The listing builds one solid part. Answer for the finished solid, in the listing's coordinates (mm). Face numbers are marked on the shaded views. Give positions to 0.01 mm unless a question says otherwise; leave off trailing zeros. Loops run counter-clockwise (first coordinate to the right, second up) from the corner with the lowest first, then second, coordinate; pieces in that order, holes last. Notation, with made-up numbers: M 67.25,-27.5 L 72.25,-27.5 A23 cw 72.25,6.5 Z; hole C 31,48.5 d11. An arc over 180 degrees is marked long. Return JSON: item names as keys, results as strings.
from build123d import *

# Parameters (mm, degrees)
BOSS_EXTRUDE1_DEPTH      = 82
BOSS_EXTRUDE1_DEPTH_BACK = 0.001
SKETCH2_W                = 480
SKETCH2_H                = 80
CUT_EXTRUDE2_DEPTH       = 82
SKETCH3_W                = 20
SKETCH3_H                = 52
SKETCH3_W_2              = 10
SKETCH3_H_2              = 82
BOSS_EXTRUDE3_DEPTH      = 30
SKETCH4_R                = 2.1
CUT_EXTRUDE3_DEPTH       = 618
SKETCH5_W                = 460.000000001
SKETCH5_H                = 31
CUT_EXTRUDE4_DEPTH       = 42
SKETCH6_R                = 2.1
CUT_EXTRUDE5_DEPTH       = 10


with BuildPart() as part:
    # Sketch1 → Boss-Extrude1 (new body, two sides)
    with BuildSketch(Plane(origin=(0, 0, 0), x_dir=(1, 0, 0), z_dir=(0, 1, 0))) as boss_extrude1_sk:
        Polygon((10, -82), (10, -52), (0, -52), (0, 0), (510, 0), (510, -82), (500, -82), (500, -52), (20, -52), (20, -82), align=None)
    extrude(amount=BOSS_EXTRUDE1_DEPTH)
    extrude(boss_extrude1_sk.sketch, amount=-BOSS_EXTRUDE1_DEPTH_BACK)

    # Sketch2 → Cut-Extrude2 (cut)
    with BuildSketch(Plane.XY):
        with Locations((260, 39.999)):
            Rectangle(SKETCH2_W, SKETCH2_H)
    extrude(amount=CUT_EXTRUDE2_DEPTH, mode=Mode.SUBTRACT)

    # Sketch3 → Boss-Extrude3 (add)
    with BuildSketch(Plane(origin=(0, 0, 0), x_dir=(1, 0, 0), z_dir=(0, 1, 0))):
        with Locations((10, -26)):
            Rectangle(SKETCH3_W, SKETCH3_H)
        with Locations((505, -41)):
            Rectangle(SKETCH3_W_2, SKETCH3_H_2)
    extrude(amount=-BOSS_EXTRUDE3_DEPTH)

    # Sketch4 → Cut-Extrude3 (cut)
    with BuildSketch(Plane(origin=(510, 0, 0), x_dir=(0, 0, -1), z_dir=(1, 0, 0))):
        with Locations((-67, -14.051)):
            Circle(SKETCH4_R)
        with Locations((-19.50000001, -14.05)):
            Circle(SKETCH4_R)
    extrude(amount=-CUT_EXTRUDE3_DEPTH, mode=Mode.SUBTRACT)

    # Sketch5 → Cut-Extrude4 (cut)
    with BuildSketch(Plane(origin=(0, 82, 0), x_dir=(1, 0, 0), z_dir=(0, 1, 0))):
        with Locations((255.200000001, -26)):
            Rectangle(SKETCH5_W, SKETCH5_H)
    extrude(amount=-CUT_EXTRUDE4_DEPTH, mode=Mode.SUBTRACT)

    # Sketch6 → Cut-Extrude5 (cut)
    with BuildSketch(Plane(origin=(20, 0, 0), x_dir=(0, 0, -1), z_dir=(1, 0, 0))):
        with Locations((-67, 11.349)):
            Circle(SKETCH6_R)
        with Locations((-60.65, 17.699)):
            Circle(SKETCH6_R)
        with Locations((-73.35, 17.699)):
            Circle(SKETCH6_R)
        with Locations((-73.35, 4.999)):
            Circle(SKETCH6_R)
        with Locations((-60.65, 4.999)):
            Circle(SKETCH6_R)
    extrude(amount=-CUT_EXTRUDE5_DEPTH, mode=Mode.SUBTRACT)


solid = part.part
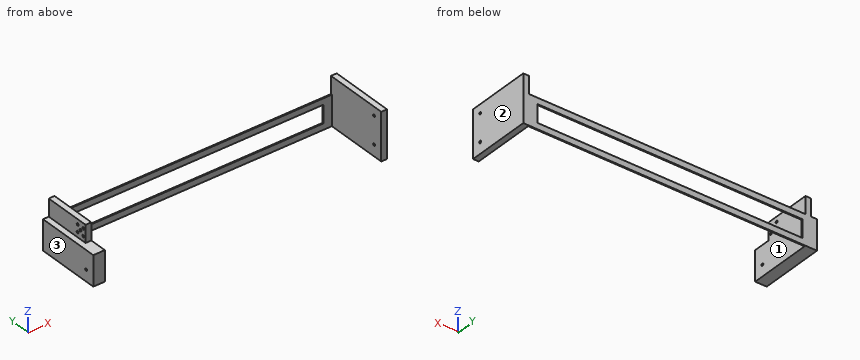
(1) Determine the mould class of the marked faces 1, 2 and 3 for opening direction X: released by +X, released by -X, zero draft, split by the parting line, or undercut.
Values follow:
{"face 1": "undercut", "face 2": "released by +X", "face 3": "released by -X"}
(2) Straight lines are drawn through the part: line 1 along X through (y, z) = (-3.5, 42); line 2 along X through (y, z) = (33.5, 57); line 3 along Y through (x, z) = (15.5, 73.35). For each, find the intervals that lie inside material, in ascending order.
Values follow:
{"line 1": "0 to 20, 500 to 510", "line 2": "10 to 20, 500 to 510", "line 3": "0 to 2.9, 7.1 to 15.6, 19.8 to 82"}
(3) The part is cut by section B-B (x = 79). Determine the outline of the cut face in (y, z).
Values follow:
{"outline": "M 80,0 L 82,0 L 82,10.5 L 80,10.5 Z; M 80,41.5 L 82,41.5 L 82,52 L 80,52 Z"}
(4) Given pin 1 (5 mm diameter, centred on x = 16, z = 64, fed in from -Y); pin 2 (5.5 mm diameter, centred on y = 4.999, z = 73.35, fed in from -X); pin 3 (5.5 mm diameter, centred on y = -14.051, z = 67, fed in from -X), each flat-ended and moving along its own axis, determine where each tip first touches the part or whether it passes through.
Values follow:
{"pin 1": "y = 0", "pin 2": "x = 10", "pin 3": "x = 500"}
(5) The part is cut by section A-A (y = 39). Determine the outline of the cut face in (x, z).
Values follow:
{"outline": "M 0,0 L 20,0 L 20,82 L 10,82 L 10,52 L 0,52 Z; M 500,0 L 510,0 L 510,82 L 500,82 Z"}
